Source: CAD feature listing. Evaluate the final solid. Frame: model axes, mm. A direction names the side the tool comes from. Give positions to 0.01 mm unless a question says otherwise; leave off trailing zeros. Loops run counter-clockwise (first coordinate to the right, second up) from the corner with the lowest first, then second, coordinate; pieces in that order, holes last. Notation, with made-up numbers: M 50,68 L 83,68 A20 ccw 83,101 Z; hole C 4.5,61 d6. An arc over 180 degrees is marked long. Put each result on its own line as item: value.
from build123d import *

# Parameters (mm, degrees)
SKETCH1_R                                           = 60
BOSS_EXTRUDE1_DEPTH                                 = 8
SKETCH2_R                                           = 4.975
SKETCH2_R_2                                         = 2.05
CUT_EXTRUDE1_DEPTH                                  = 86.229103011
CIRPATTERN1_COUNT                                   = 4
SKETCH4_R                                           = 34.5
SKETCH4_R_2                                         = 30.5
BOSS_EXTRUDE2_DEPTH                                 = 12.5
SKETCH5_R                                           = 20
BOSS_EXTRUDE3_DEPTH                                 = 1
SKETCH6_R                                           = 17.5
BOSS_EXTRUDE4_DEPTH                                 = 18
SKETCH7_R                                           = 7.5
CUT_EXTRUDE2_DEPTH                                  = 90.044932478
BOSS_EXTRUDE6_START                                 = -2
SKETCH9_R                                           = 4.975
BOSS_EXTRUDE6_DEPTH                                 = 2
SKETCH10_R                                          = 4.975
BOSS_EXTRUDE7_DEPTH                                 = 3
CHAMFER2_START                                      = -3.006253442
CHAMFER2_DEPTH                                      = 0.006253442
CHAMFER2_START_2                                    = -7.5000001
CHAMFER2_2_DEPTH                                    = 4.493746658
CHAMFER2_3_ANGLE                                    = 16.582247
CIRPATTERN2_COUNT                                   = 4
CSK_FOR_M4_COUNTERSUNK_FLAT_HEAD_SCREW1_D           = 3.6
CSK_FOR_M4_COUNTERSUNK_FLAT_HEAD_SCREW1_CSINK_D     = 9.1
CSK_FOR_M4_COUNTERSUNK_FLAT_HEAD_SCREW1_CSINK_ANGLE = 90
BOSS_EXTRUDE8_DEPTH                                 = 12.5


with BuildPart() as part:
    # Sketch1 → Boss-Extrude1 (new body)
    with BuildSketch(Plane(origin=(0, 0, 0), x_dir=(1, 0, 0), z_dir=(0, 1, 0))):
        with Locations(Location((0, 0, 0), (0, 0, 270))):
            Circle(SKETCH1_R)
    extrude(amount=BOSS_EXTRUDE1_DEPTH)

    # Sketch2 → Cut-Extrude1 (cut, through all)
    with BuildSketch(Plane(origin=(0, 8, 0), x_dir=(1, 0, 0), z_dir=(0, 1, 0))):
        with Locations(Location((-33.587572106, -33.587572106, 0), (0, 0, 270))):
            Circle(SKETCH2_R)
        with Locations(Location((-43.487067043, -23.68807717, 0), (0, 0, 270))):
            Circle(SKETCH2_R_2)
        with Locations(Location((-23.68807717, -43.487067043, 0), (0, 0, 270))):
            Circle(SKETCH2_R_2)
        with Locations(Location((0, -49.52, 0), (0, 0, 270))):
            Circle(SKETCH2_R_2)
    cut_extrude1 = extrude(amount=-CUT_EXTRUDE1_DEPTH, mode=Mode.SUBTRACT)

    # CirPattern1: Cut-Extrude1 ×4 about axis
    cirpattern1_axis = Axis((0, 0, 0), (0, 1, 0))
    for i in range(1, CIRPATTERN1_COUNT):
        add(cut_extrude1.rotate(cirpattern1_axis, i * 360 / CIRPATTERN1_COUNT), mode=Mode.SUBTRACT)

    # Sketch4 → Boss-Extrude2 (add)
    with BuildSketch(Plane.XZ):
        with Locations(Location((0, 0, 0), (0, 0, 90))):
            Circle(SKETCH4_R)
        with Locations(Location((0, 0, 0), (0, 0, 270))):
            Circle(SKETCH4_R_2, mode=Mode.SUBTRACT)
    extrude(amount=BOSS_EXTRUDE2_DEPTH)

    # Sketch5 → Boss-Extrude3 (add)
    with BuildSketch(Plane.XZ):
        with Locations(Location((0, 0, 0), (0, 0, 90))):
            Circle(SKETCH5_R)
    extrude(amount=BOSS_EXTRUDE3_DEPTH)

    # Sketch6 → Boss-Extrude4 (add)
    with BuildSketch(Plane.XZ.offset(1)):
        with Locations(Location((0, 0, 0), (0, 0, 270))):
            Circle(SKETCH6_R)
    extrude(amount=BOSS_EXTRUDE4_DEPTH)

    # Sketch7 → Cut-Extrude2 (cut, through all)
    with BuildSketch(Plane.XZ.offset(19)):
        with Locations(Location((0, 0, 0), (0, 0, 270))):
            Circle(SKETCH7_R)
    extrude(amount=-CUT_EXTRUDE2_DEPTH, mode=Mode.SUBTRACT)

    # Sketch9 → Boss-Extrude6 (add)
    with BuildSketch(Plane.XZ.offset(BOSS_EXTRUDE6_START)):
        with Locations(Location((-33.587572106, -33.587572106, 0), (0, 0, 180))):
            Circle(SKETCH9_R)
        with Locations(Location((-33.587572106, 33.587572106, 0), (0, 0, 90))):
            Circle(SKETCH9_R)
        with Locations((33.587572106, 33.587572106)):
            Circle(SKETCH9_R)
        with Locations(Location((33.587572106, -33.587572106, 0), (0, 0, 270))):
            Circle(SKETCH9_R)
    extrude(amount=BOSS_EXTRUDE6_DEPTH)

    # Sketch10 → Boss-Extrude7 (add)
    with BuildSketch(Plane.XZ):
        with BuildLine():
            Line((20.6223527, -27.658065173), (30.06971587, -37.105428343))
            ThreePointArc((30.06971587, -37.105428343), (30.06971587, -30.06971587), (37.105428343, -30.06971587))
            Line((37.105428343, -30.06971587), (27.658065173, -20.6223527))
            ThreePointArc((27.658065173, -20.6223527), (24.395183951, -24.395183951), (20.6223527, -27.658065173))
        make_face()
        with Locations(Location((33.587572106, -33.587572106, 0), (0, 0, 270))):
            Circle(SKETCH10_R)
    boss_extrude7 = extrude(amount=BOSS_EXTRUDE7_DEPTH)

    # Chamfer2: read off the stored shape, not the designer's step
    # Chamfer2 outline → Chamfer2 (add)
    with BuildSketch(Plane(origin=(0, 0, 0), x_dir=(1, 0, 0), z_dir=(0, 1, 0)).offset(CHAMFER2_START)):
        with BuildLine():
            ThreePointArc((37.105428343, 30.06971587), (37.105428343, 37.105428343), (30.06971587, 37.105428343))
            Line((30.06971587, 37.105428343), (20.6223527, 27.658065173))
            ThreePointArc((20.6223527, 27.658065173), (24.395183951, 24.395183951), (27.658065173, 20.6223527))
            Line((27.658065173, 20.6223527), (37.105428343, 30.06971587))
        make_face()
    chamfer2 = extrude(amount=CHAMFER2_DEPTH)

    # Chamfer2 2 outline → Chamfer2 2 (add)
    with BuildSketch(Plane(origin=(0, 0, 0), x_dir=(1, 0, 0), z_dir=(0, 1, 0)).offset(CHAMFER2_START_2)):
        with BuildLine():
            ThreePointArc((37.105428343, 30.06971587), (37.105428343, 37.105428343), (30.06971587, 37.105428343))
            Line((30.06971587, 37.105428343), (20.6223527, 27.658065173))
            ThreePointArc((20.6223527, 27.658065173), (24.395183951, 24.395183951), (27.658065173, 20.6223527))
            Line((27.658065173, 20.6223527), (37.105428343, 30.06971587))
        make_face()
    chamfer2_2 = extrude(amount=CHAMFER2_2_DEPTH)

    # Chamfer2 3 outline → Chamfer2 3 (revolve, cut)
    with BuildSketch(Plane(origin=(0, 0, 0), x_dir=(0.801683048491221, 0, -0.597749353627273), z_dir=(0.597749353627273, 0, 0.801683048491221))):
        Polygon((52.475017897, -3.006245526), (34.5, -7.5), (52.475, -7.5000001), align=None)
    chamfer2_3 = revolve(axis=Axis((0, 0, 0), (0, 1, 0)), revolution_arc=CHAMFER2_3_ANGLE, mode=Mode.SUBTRACT)

    # CirPattern2: Boss-Extrude7, Chamfer2, Chamfer2 2, Chamfer2 3 ×4 about axis
    cirpattern2_axis = Axis((0, 0, 0), (0, 1, 0))
    add([boss_extrude7.rotate(cirpattern2_axis, i * 360 / CIRPATTERN2_COUNT) for i in range(1, CIRPATTERN2_COUNT)])
    add([chamfer2.rotate(cirpattern2_axis, i * 360 / CIRPATTERN2_COUNT) for i in range(1, CIRPATTERN2_COUNT)])
    add([chamfer2_2.rotate(cirpattern2_axis, i * 360 / CIRPATTERN2_COUNT) for i in range(1, CIRPATTERN2_COUNT)])
    add([chamfer2_3.rotate(cirpattern2_axis, i * 360 / CIRPATTERN2_COUNT) for i in range(1, CIRPATTERN2_COUNT)], mode=Mode.SUBTRACT)

    # CSK for M4 Countersunk Flat Head Screw1 (through all)
    with Locations(Plane(origin=(0, 8, -12.5), x_dir=(0, 0, 1), z_dir=(0, 1, 0))):
        with Locations((0, 0), (12.5, 12.5), (25, 0), (12.5, -12.5)):
            CounterSinkHole(CSK_FOR_M4_COUNTERSUNK_FLAT_HEAD_SCREW1_D / 2, CSK_FOR_M4_COUNTERSUNK_FLAT_HEAD_SCREW1_CSINK_D / 2, counter_sink_angle=CSK_FOR_M4_COUNTERSUNK_FLAT_HEAD_SCREW1_CSINK_ANGLE)

    # Sketch13 → Boss-Extrude8 (add)
    with BuildSketch(Plane.XZ):
        with BuildLine():
            Line((-11.79321147, -32.421754475), (-12.732901193, -35.928724264))
            ThreePointArc((-12.732901193, -35.928724264), (-10.611580849, -39.602958878), (-6.937346235, -37.481638534))
            Line((-6.937346235, -37.481638534), (-5.997656512, -33.974668745))
            ThreePointArc((-5.997656512, -33.974668745), (-8.929257056, -33.324441007), (-11.79321147, -32.421754475))
        make_face()
    extrude(amount=BOSS_EXTRUDE8_DEPTH)


solid = part.part
1. Section query D-D (z = -49.52). Output: boundary loops of the cut face in (x, y).
Found:
outline: M -33.88,0 L -2.05,0 L -2.05,8 L -33.88,8 Z; M 2.05,0 L 33.88,0 L 33.88,8 L 2.05,8 Z
2. Draft query along Z for faces 1 (the flat face through (25.28, -2.969, 32.316)), 2 (the cylindrical face through (-29.921, 5.042, -30.225)), 3 (the flat face through (-12, 8, 12)). Return one class per face: pulls with the +Z half, pulls with the -Z half, needs draft (parallel to the pull), parting line crosses it, or undercut.
Found:
face 1: pulls with the +Z half
face 2: undercut
face 3: needs draft
3. Contact query for flat-ended pins moving along their axis: P1, Ø12, axis at x = 0, z = 0, coming from the +Y side; P2, Ø6, axis at x = 3.5, y = -2.5, coming from the -Z side; P3, Ø3, axis at x = -31.5, z = -31, coming from the +Y side; P4, Ø4, axis at x = -31, z = 11.5, coming from the -Y side. Output: stop coordinate, or through.
Found:
P1: through
P2: z = -59.97
P3: y = 2
P4: y = -12.5
4. Section query B-B (z = -12.5). Output: boundary loops of the cut face in (x, y), plus the area to 3 significant figures.
Found:
outline: M -58.68,0 L -32.16,0 L -32.16,-12.5 L -27.82,-12.5 L -27.82,0 L -15.61,0 L -15.61,-1 L -12.25,-1 L -12.25,-19 L -1.8,-19 L -1.8,5.25 L -4.55,8 L -58.68,8 Z; M 1.8,-19 L 12.25,-19 L 12.25,-1 L 15.61,-1 L 15.61,0 L 27.82,0 L 27.82,-12.5 L 32.16,-12.5 L 32.16,0 L 58.68,0 L 58.68,8 L 4.55,8 L 1.8,5.25 Z
area: 1,410 mm^2
5. Section query C-C (x = 0). State how many separate pieces and enclosed holes the cut face has, plus the area to 3 significant figures.
Found:
separate pieces: 6
enclosed holes: 0
area: 1,050 mm^2
6. Material intervals for line 1 (X direction, y = -5.25, z = 5); line 2 (Z direction, x = 45, y = 4.5); line 3 (X direction, y = -2.5, z = -15), sorted ascending. Write a range as from..to.
Found:
line 1: -34.14..-30.09, -16.77..-5.59, 5.59..16.77, 30.09..34.14
line 2: -39.69..-25.07, -22.3..22.3, 25.07..39.69
line 3: -31.07..-26.56, -9.01..9.01, 26.56..31.07
7. Section query A-A (x = 12.5). Output: boundary loops of the cut face in (y, z).
Found:
outline: M -19,-12.25 L -1,-12.25 L -1,-15.61 L 0,-15.61 L 0,-27.82 L -12.5,-27.82 L -12.5,-32.16 L 0,-32.16 L 0,-58.68 L 8,-58.68 L 8,-4.55 L 5.25,-1.8 L -19,-1.8 Z; M -19,1.8 L 5.25,1.8 L 8,4.55 L 8,58.68 L 0,58.68 L 0,32.16 L -12.5,32.16 L -12.5,27.82 L 0,27.82 L 0,15.61 L -1,15.61 L -1,12.25 L -19,12.25 Z
8. Access query for faces 4 (the flat face through (-32.316, -2.969, 25.28)), 5 (the cylindrical face through (-10.648, -9.874, 13.887)), 6 (the flat face through (-25.28, -2.864, 32.316)), 7 (the flat face through (25.412, -2.969, -32.448)), 8 (the flat face through (-34, 2, 34)). Directions: +Z, -Z, +X, -X, +Y, -Y. A direction counts if a zero-diameter tool reaches every point of the face in a straight line with its end or side. Return the directions, or none.
Found:
face 4: -X, -Y
face 5: -Y
face 6: +Z, -Y
face 7: -Z, -Y
face 8: +Y
